Design review of the part built by this model. Coordinates are the model's own, in mm. Face numbers are marked on the shaded views. A direction names the side the tool comes from. Coordinates: 2 decimals unless noted, no trailing zeros. Write each loop counter-clockwise with the first axis right and the second up, starting at its lowest first coordinate (ties: lowest second). Pieces come first, ordered by that corner, then holes.
Q1. Machinability: for the marked faces 1, 2, 3, 4 and 5, which of the approach directions +Z, -Z, +X, -X, +Y, -Y give a long, thin tool a straight path to every point of the face, cutting with its end or side? Answer none if there is none.
Q2. For probe 1 along Z at (x, y) = (9, -72); probe 2 along Z at (x, y) = (25, -32.5); probe 3 along Y at (x, z) = (-54, -14), list the stretches that pass through material, from the lowest coordinate up.
Q3. Take a section at D-D (y = -63.5). Give the boundary of the cut face in (x, z).
Q4. Take a section at B-B (z = 65). Give the boundary of the cut face in (x, y), and give its area (3 significant figures).
Q5. Take a section at A-A (y = -77). Give the boundary of the cut face in (x, z).
Q6. Insertion check: pin 1 (1.5 mm diameter, centred on y = -23.5, z = -13, fed in from +X); pin 2 (2.5 mm diameter, centred on x = 3, y = -23, fed in from +Z); pin 3 (12 mm diameter, centred on x = 55.5, y = -46.5, fed in from -Z); pin 4 (1.9 mm diameter, centred on x = -76, y = -17, fed in from -Z). Each pin has a flat end and moves straight along its axis. Give the tip position at first contact, or say it passes through.
Q7. Take a section at C-C (x = 0). Give the boundary of the cut face in (y, z).
Q8. Mouldability with a two-part tool opening along Z and no side actions: class the marked faces 6, 7, 8 and 9 as pulls with the +Z half, pulls with the -Z half, needs draft (parallel to the pull), parting line crosses it, or undercut.
```python
from build123d import *

# Parameters (mm, degrees)
F1_W      = 151.3319835067
F1_H      = 147.9758322239
F2_DEPTH  = 20.066
F3_W      = 75.2840787172
F3_H      = 76.1998519301
F3_H_2    = 71.7759802938
F3_W_2    = 76.0479047894
F4_DEPTH  = 0.254
F5_R      = 49.1952148829
F6_DEPTH  = 25.4
F7_R      = 49.1952148829
F8_DEPTH  = 25.4
F10_R     = 3.1853850864
F10_R_2   = 3.4787314223
F10_R_3   = 3.5581054838
F10_R_4   = 2.8783548202
F10_R_5   = 2.4598319218
F10_R_6   = 3.3699911713
F10_R_7   = 3.478728155
F10_R_8   = 3.1114703305
F10_R_9   = 3.1412466135
F10_R_10  = 3.2433066159
F10_R_11  = 3.5711592921
F10_R_12  = 2.6246103999
F10_R_13  = 3.3699920988
F10_R_14  = 3.4787300337
F10_R_15  = 3.4787284
F10_R_16  = 3.4111759436
F10_R_17  = 2.7289404217
F10_R_18  = 3.3002128489
F10_R_19  = 4.0130328481
F10_R_20  = 3.4787270114
F11_DEPTH = 25.4
F0_W      = 2.5908052921
F0_H      = 16.4592005312
F0_W_2    = 4.267193377
F0_H_2    = 17.0687958598
F0_H_3    = 16.7640019208
F0_W_3    = 3.8100033998
F0_H_4    = 16.154400073
F0_W_4    = 18.8976023346
F0_H_5    = 2.438403666
F0_H_6    = 0.6095990539
F0_H_7    = 16.7640000582
F0_W_5    = 34.7471982241
F0_H_8    = 18.592800945
F0_W_6    = 17.0688033104
F0_W_7    = 4.2672008276
F0_W_8    = 21.3360004127
F0_H_9    = 3.0480027199
F0_W_9    = 2.8956010938
F12_DEPTH = 25.4
F13_W     = 115.3296120465
F13_H     = 117.7704520524
F14_DEPTH = 50.8
F15_R     = 10.1970754687
F15_R_2   = 10.573540908
F15_R_3   = 12.1455637772
F16_DEPTH = 25.4
F17_W     = 22.5777532905
F17_H     = 16.4756593294
F17_W_2   = 23.7981723621
F17_H_2   = 16.7807638645
F17_W_3   = 24.4083832949
F17_H_3   = 20.1369160786
F18_DEPTH = 25.4


with BuildPart() as f2:
    # F1 (on Front) → F2 (new body)
    with BuildSketch(Plane.XZ):
        with Locations((0.3819130361, 2.2119358182)):
            Rectangle(F1_W, F1_H)
    extrude(amount=F2_DEPTH)

    # F3 (on face) → F4 (join)
    with BuildSketch(Plane.XZ.offset(20.066)):
        with Locations((-37.6420393586, 38.0999259651)):
            Rectangle(F3_W, F3_H)
        with Locations((-37.6420393586, -35.8879901469)):
            Rectangle(F3_W, F3_H_2)
        with Locations((38.0239523947, -35.8879901469)):
            Rectangle(F3_W_2, F3_H_2)
        with Locations((38.0239523947, 38.0999259651)):
            Rectangle(F3_W_2, F3_H)
    extrude(amount=F4_DEPTH)

    # F5 (on face) → F6 (join)
    with BuildSketch(Plane.XZ.offset(20.32)):
        Circle(F5_R)
    extrude(amount=F6_DEPTH)

    # F7 (on face) → F8 (join)
    with BuildSketch(Plane.XZ.offset(45.72)):
        Circle(F7_R)
    extrude(amount=F8_DEPTH)

    # F10 (on Front) → F11 (join)
    with BuildSketch(Plane.XZ):
        with Locations((45.2323183417, 56.9782480597)):
            Circle(F10_R)
        with Locations((18.0779919028, 56.6731393337)):
            Circle(F10_R_2)
        with Locations((-8.771231398, 56.6731393337)):
            Circle(F10_R_3)
        with Locations((-31.6540896893, 56.6731393337)):
            Circle(F10_R_4)
        with Locations((-49.3501722813, 56.6731393337)):
            Circle(F10_R_5)
        with Locations((45.8425283432, 20.0605653226)):
            Circle(F10_R_6)
        with Locations((18.0779919028, 19.1452521831)):
            Circle(F10_R_7)
        with Locations((-8.1610223278, 20.0605653226)):
            Circle(F10_R_8)
        with Locations((-28.9081465453, 19.1452521831)):
            Circle(F10_R_9)
        with Locations((-52.4012185633, 18.2299371809)):
            Circle(F10_R_10)
        with Locations((46.4527383447, -12.8907542676)):
            Circle(F10_R_11)
        with Locations((19.6035150439, -12.5856492668)):
            Circle(F10_R_12)
        with Locations((-8.4661273286, -12.5856492668)):
            Circle(F10_R_13)
        with Locations((-31.0438796878, -13.1958574057)):
            Circle(F10_R_14)
        with Locations((-52.4012185633, -12.2805442661)):
            Circle(F10_R_15)
        with Locations((46.4527383447, -45.8420701325)):
            Circle(F10_R_16)
        with Locations((20.5188300461, -45.536968857)):
            Circle(F10_R_17)
        with Locations((-10.2967554703, -46.75738886)):
            Circle(F10_R_18)
        with Locations((-31.6540896893, -47.0624901354)):
            Circle(F10_R_19)
        with Locations((-52.4012185633, -47.3675951362)):
            Circle(F10_R_20)
    extrude(amount=F11_DEPTH)

    # F0 (on Front) → F12 (join)
    with BuildSketch(Plane.XZ):
        with Locations((-75.2094015479, 37.0332021266)):
            Rectangle(F0_W, F0_H)
        with Locations((-71.7804022133, 53.7972003222)):
            Rectangle(F0_W_2, F0_H_2)
        with Locations((-71.7804022133, 37.0332021266)):
            Rectangle(F0_W_2, F0_H)
        Polygon((-73.9139989018, 72.9995965958), (-73.9139989018, 62.3315982521), (-69.6468055248, 62.3315982521), (-69.6468055248, 68.7323957682), (-57.6071999967, 68.7323957682), (-57.6071999967, 72.9995965958), align=None)
        Polygon((-75.1331970096, 62.3315982521), (-73.9139989018, 62.3315982521), (-73.9139989018, 72.9995965958), (-57.6071999967, 72.9995965958), (-57.6071999967, 75.1332044601), (-36.271199584, 75.1332044601), (-36.271199584, 72.9995965958), (-4.1148010641, 72.9995965958), (-4.1148010641, 75.4380002618), (-75.1331970096, 75.4380002618), align=None)
        with Locations((-71.7804022133, 20.4216009006)):
            Rectangle(F0_W_2, F0_H_3)
        with Locations((-75.8190006018, 3.9623999037)):
            Rectangle(F0_W_3, F0_H_4)
        with Locations((-71.7804022133, 3.9623999037)):
            Rectangle(F0_W_2, F0_H_4)
        with Locations((-71.7804022133, -12.1920001693)):
            Rectangle(F0_W_2, F0_H_4)
        with Locations((5.3340001032, 74.2187984288)):
            Rectangle(F0_W_4, F0_H_5)
        with Locations((5.3340001032, 75.7427997887)):
            Rectangle(F0_W_4, F0_H_6)
        with Locations((-75.2094015479, -28.6512002349)):
            Rectangle(F0_W, F0_H_7)
        with Locations((-71.7804022133, -28.6512002349)):
            Rectangle(F0_W_2, F0_H_7)
        with Locations((32.1564003825, 74.2187984288)):
            Rectangle(F0_W_5, F0_H_5)
        with Locations((-71.7804022133, -46.3296007365)):
            Rectangle(F0_W_2, F0_H_8)
        with Locations((58.0644011497, 74.2187984288)):
            Rectangle(F0_W_6, F0_H_5)
        Polygon((-73.9139989018, -68.4275999665), (-73.9139989018, -55.626001209), (-76.504804194, -55.626001209), (-76.504804194, -71.4756026864), (-57.6071999967, -71.4756026864), (-57.6071999967, -68.4275999665), align=None)
        Polygon((-69.6468055248, -55.626001209), (-73.9139989018, -55.626001209), (-73.9139989018, -68.4275999665), (-57.6071999967, -68.4275999665), (-57.6071999967, -63.2460042834), (-69.6468055248, -63.2460042834), align=None)
        Polygon((75.7427960634, 75.4380002618), (66.5988028049, 75.4380002618), (66.5988028049, 72.9995965958), (73.304399848, 72.9995965958), (73.304399848, 62.3315982521), (75.7427960634, 62.3315982521), align=None)
        with Locations((71.1707994342, 53.7972003222)):
            Rectangle(F0_W_7, F0_H_2)
        with Locations((71.1707994342, 37.0332021266)):
            Rectangle(F0_W_7, F0_H)
        Polygon((73.304399848, 72.9995965958), (66.5988028049, 72.9995965958), (66.5988028049, 68.7323957682), (69.0371990204, 68.7323957682), (69.0371990204, 62.3315982521), (73.304399848, 62.3315982521), align=None)
        with Locations((-46.9391997904, -69.9516013265)):
            Rectangle(F0_W_8, F0_H_9)
        with Locations((74.7522003949, 37.0332021266)):
            Rectangle(F0_W_9, F0_H)
        with Locations((71.1707994342, 20.4216009006)):
            Rectangle(F0_W_7, F0_H_3)
        Polygon((-4.1148010641, -68.4275999665), (-36.271199584, -68.4275999665), (-36.271199584, -71.4756026864), (49.5299994946, -71.4756026864), (49.5299994946, -68.4275999665), (14.7828012705, -68.4275999665), (14.7828012705, -70.8660036325), (-4.1148010641, -70.8660036325), align=None)
        with Locations((71.1707994342, 3.9623999037)):
            Rectangle(F0_W_7, F0_H_4)
        with Locations((74.7522003949, 3.9623999037)):
            Rectangle(F0_W_9, F0_H_4)
        with Locations((71.1707994342, -12.1920001693)):
            Rectangle(F0_W_7, F0_H_4)
        with Locations((58.0644011497, -69.9516013265)):
            Rectangle(F0_W_6, F0_H_9)
        with Locations((71.1707994342, -28.6512002349)):
            Rectangle(F0_W_7, F0_H_7)
        Polygon((66.5988028049, -68.4275999665), (66.5988028049, -71.4756026864), (76.2000009418, -71.4756026864), (76.2000009418, -55.626001209), (73.304399848, -55.626001209), (73.304399848, -68.4275999665), align=None)
        with Locations((74.7522003949, -28.6512002349)):
            Rectangle(F0_W_9, F0_H_7)
        with Locations((71.1707994342, -46.3296007365)):
            Rectangle(F0_W_7, F0_H_8)
        Polygon((66.5988028049, -63.2460042834), (66.5988028049, -68.4275999665), (73.304399848, -68.4275999665), (73.304399848, -55.626001209), (69.0371990204, -55.626001209), (69.0371990204, -63.2460042834), align=None)
    extrude(amount=F12_DEPTH)

    # F13 (on Front) → F14 (join)
    with BuildSketch(Plane.XZ):
        with Locations((0.0768061727, 3.5849083215)):
            Rectangle(F13_W, F13_H)
    extrude(amount=F14_DEPTH)

    # F15 (on face) → F16 (join)
    with BuildSketch(Plane.XZ.offset(71.12)):
        with Locations((-21.2805289775, 15.4839931056)):
            Circle(F15_R)
        with Locations((18.993306905, 14.5686790347)):
            Circle(F15_R_2)
        with Locations((0, -20.2132686973)):
            Circle(F15_R_3)
    extrude(amount=F16_DEPTH)

    # F17 (on face) → F18 (join)
    with BuildSketch(Plane.XZ.offset(71.12)):
        with Locations((-21.5856330469, 15.1788888033)):
            Rectangle(F17_W, F17_H)
        with Locations((19.2984095775, 14.4161265343)):
            Rectangle(F17_W_2, F17_H_2)
        with Locations((0.0768071041, -20.8234782331)):
            Rectangle(F17_W_3, F17_H_3)
    extrude(amount=F18_DEPTH)


solid = f2.part
```
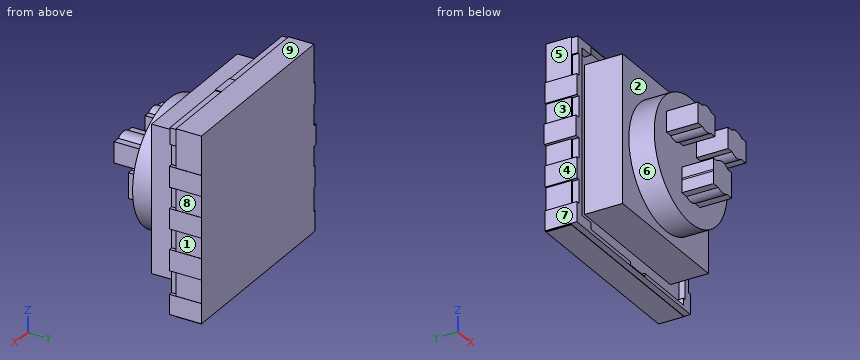
Response:
1. face 1: +X, +Y, -Y
1. face 2: -Y
1. face 3: -X, +Y, -Y
1. face 4: -Z, -X, +Y, -Y
1. face 5: +Z, -X, +Y, -Y
2. probe 1: z = -30.89 to -10.76, 6.03 to 22.81
2. probe 2: z = -55.3 to 62.47
2. probe 3: y = -50.8 to 0
3. outline: circle Ø98.39 at (0, 0)
4. outline: (-75.28, -20.32) - (-75.13, -20.32) - (-75.13, -25.4) - (-69.65, -25.4) - (-69.65, -20.32) - (69.04, -20.32) - (69.04, -25.4) - (75.74, -25.4) - (75.74, -20.32) - (76.05, -20.32) - (76.05, 0) - (-75.28, 0) - close
4. area: 3,140 mm2
5. outline: (-32.87, 6.94) - (-26.85, 6.94) arc R10.2 ccw to (-15.71, 6.94) - (-10.3, 6.94) - (-10.3, 23.42) - (-14.87, 23.42) arc R10.2 ccw to (-27.69, 23.42) - (-32.87, 23.42) - close; (-12.13, -30.89) - (-5.79, -30.89) arc R12.15 ccw to (5.79, -30.89) - (12.28, -30.89) - (12.28, -10.76) - (7.62, -10.76) arc R12.15 ccw to (-7.62, -10.76) - (-12.13, -10.76) - (-12.13, -19.55) arc R12.15 ccw to (-12.13, -20.88) - close; (7.4, 6.03) - (12.76, 6.03) arc R10.57 ccw to (25.22, 6.03) - (31.2, 6.03) - (31.2, 22.81) - (25.62, 22.81) arc R10.57 ccw to (12.36, 22.81) - (7.4, 22.81) - close
6. pin 1: stops at x = 73.3
6. pin 2: stops at z = 76.05
6. pin 3: stops at z = -55.3
6. pin 4: stops at z = -71.78
7. outline: (-96.52, -32.36) - (-71.12, -32.36) - (-71.12, -49.2) - (-50.8, -49.2) - (-50.8, -55.3) - (-20.32, -55.3) - (-20.32, -70.87) - (-25.4, -70.87) - (-25.4, -71.48) - (-20.32, -71.48) - (-20.32, -71.78) - (0, -71.78) - (0, 76.2) - (-20.32, 76.2) - (-20.32, 76.05) - (-25.4, 76.05) - (-25.4, 73) - (-20.32, 73) - (-20.32, 62.47) - (-50.8, 62.47) - (-50.8, 49.2) - (-71.12, 49.2) - (-71.12, -8.07) - (-96.52, -8.07) - close
8. face 6: parting line crosses it
8. face 7: needs draft
8. face 8: undercut
8. face 9: pulls with the +Z half
